Here's how the part is built. I have some questions about the finished solid (model axes, mm). A direction names the side the tool comes from. Give positions to 0.01 mm unless a question says otherwise; leave off trailing zeros. Loops run counter-clockwise (first coordinate to the right, second up) from the corner with the lowest first, then second, coordinate; pieces in that order, holes last. Notation, with made-up numbers: M 13.25,-20.75 L 33.25,-20.75 A14 cw 33.25,-10.75 Z; hole C 73,21 d6. An arc over 180 degrees is marked long. Write item = value, one per line. Start each with the question number.
Autodesk Fusion 360 part; units mm, degrees
sketch "Sketch1" plane through (0, 0, 0) normal (0, 0, 1) x (1, 0, 0)
  line L0 (0, 0) -> (0, -37.5335) construction
  line L1 (31.3, -31.3) -> (31.3, 13.7)
  line L2 (31.3, -31.3) -> (2, -2)
  line L3 (-31.3, -31.3) -> (-31.3, 13.7)
  line L4 (-31.3, -31.3) -> (-2, -2)
  line L5 (31.3, 13.7) -> (-31.3, 13.7)
  arc A0 (2, -2) -> (-2, -2) centre (0, -2) ccw
  dimension "d1" = 62.6
  dimension "d2" = 45
  dimension "d4" = 90
  dimension "d5" = 2
extrude "Extrude1" add sketch "Sketch1" along normal blind 56
sketch "Sketch2" plane through (0, 0, 0) normal (0.7071, -0.7071, 0) x (0.7071, 0.7071, 0)
  line L0 (-44.2649, 0) -> (-2.8284, 0)
  line L1 (-2.8284, 0) -> (-2.8284, 56)
  line L2 (-2.8284, 56) -> (-44.2649, 56)
  line L3 (-44.2649, 56) -> (-44.2649, 0)
  circle A0 centre (-25.8284, 41) radius 2
  circle A1 centre (-25.8284, 15) radius 2
  circle A2 centre (-25.8284, 15) radius 6.5
  circle A3 centre (-25.8284, 41) radius 6.5
  dimension "d8" = 15
  dimension "d10" = 4
  dimension "d11" = 15
  dimension "d12" = 23
  dimension "d15" = 13
extrude "Extrude2" cut sketch "Sketch2" against normal blind 61.002 contours A0 | A1
extrude "Extrude3" cut sketch "Sketch2" along normal blind 17 from surface at -30 contours A2 | A3
sketch "Sketch3" plane through (0, 13.7, 0) normal (0, 1, 0) x (-1, 0, 0)
  line L0 (-31.3, 0) -> (31.3, 0)
  line L1 (31.3, 0) -> (31.3, 56)
  line L2 (31.3, 56) -> (-31.3, 56)
  line L3 (-31.3, 56) -> (-31.3, 0)
  line L4 (0, 56) -> (0, 42.8245) construction
  circle A0 centre (-22.5, 31) radius 1.5
  circle A1 centre (22.5, 31) radius 1.5
  circle A2 centre (0, 8.5) radius 1.5
  dimension "d19" = 25
  dimension "d20" = 45
  dimension "d21" = 3
  dimension "d30" = 8.5
hole "Hole1" at (22.5, 13.7, 31) at (-22.5, 13.7, 31) at (0, 13.7, 8.5) direction (0, -1, 0) diameter 2.529 depth 25 tip angle 118
fillet "Fillet1" radius 9 4 edges at (31.3, -8.8, 56) (-31.3, -8.8, 56) (-31.3, -8.8, 0) (31.3, -8.8, 0)
mirror "Mirror1" about plane through (0, 0, 0) normal (1, 0, 0) of "Extrude2", "Extrude3"
equation "d11 = d8"
Q1. If we section it at D-D, the plane z = 24.5: List the corners of the cut face in (x, y) for me, then the cut area to 3 significant figures.
Q2. If we section it at B-B, the plane x = 0: List the corners of the cut face in (y, z) for me.
Q3. If we section it at A-A, the plane y = -27: List the corners of the cut face in (x, z) for me, then the cut area to 3 significant figures.
Q4. We'd pull the mould along X, two halves only. Please class faces 1 (the cylindrical face through (-26.2, -1.14, 15.23)), 2 (the cylindrical face through (-28.734, 6.112, 53.294)), 3 (the flat face through (0, 4, 0)), 4 (the conical face through (22.566, -11.928, 31.209)): pulls with the +X half, pulls with the -X half, needs draft (parallel to the pull), parting line crosses it, or undercut.
Q5. If I drill on line 1 along X through (y, z) = (5, 31); line 2 along Z through (x, y) = (-22.5, 5.75); line 3 along Z through (x, y) = (0, 10), over which ranges is the centre line in solid material (lowest first)?
Q6. On a 3-axis mill with a long thin cutter (end or side, diameter ignored), from which of +Z, -Z, +X, -X, +Y, -Y can I reach the whole of each face in a straight line? I mean faces 5 (the flat face through (17, -17, 28)), 6 (the cylindrical face through (22.1, 1, 32.2)), 7 (the cylindrical face through (26.2, -1.14, 40.77)). Say none if no direction works.
Q7. If we section it at C-C, the plane y = 5: List the corners of the cut face in (x, z) for me, then the cut area to 3 significant figures.
Q8. Will these pins go through, and if not, where does the flat tip stop? pin 1 (6 mm diameter, centred on x = -15.5, y = 2, fed in from -Z); pin 2 (2.5 mm diameter, centred on x = -22.5, z = 31, fed in from -Y).
Resolved:
q1.outline = M -31.3,-31.3 L -2,-2 A2 cw 2,-2 L 31.3,-31.3 L 31.3,13.7 L -31.3,13.7 Z
q1.area = 1,840 mm²
q2.outline = M 0,0 L 13.7,0 L 13.7,7.24 L 0,7.24 Z; M 0,9.76 L 13.7,9.76 L 13.7,56 L 0,56 Z
q3.outline = M -31.3,9 A9 ccw -27,1.32 L -27,54.68 A9 ccw -31.3,47 Z; M 27,1.32 A9 ccw 31.3,9 L 31.3,47 A9 ccw 27,54.68 Z
q3.area = 420 mm²
q4.face_1 = undercut
q4.face_2 = pulls with the -X half
q4.face_3 = needs draft
q4.face_4 = undercut
q5.line_1 = -31.3 to -23.76, -21.24 to 21.24, 23.76 to 31.3
q5.line_2 = 0 to 29.74, 32.26 to 56
q5.line_3 = 0 to 7.24, 9.76 to 56
q6.face_5 = +Z, -Z, -Y
q6.face_6 = +Y
q6.face_7 = none
q7.outline = M -31.3,9 A9 ccw -22.3,0 L 22.3,0 A9 ccw 31.3,9 L 31.3,47 A9 ccw 22.3,56 L -22.3,56 A9 ccw -31.3,47 Z; hole C -22.5,31 d2.53; hole C 0,8.5 d2.53; hole C 22.5,31 d2.53
q7.area = 3,420 mm²
q8.pin_1 = 0
q8.pin_2 = -23.75
